For this review, take the finished solid that the model builds, in its own axes (mm). Give positions to 0.01 mm unless a question says otherwise; leave off trailing zeros. Order: outer loops, then holes, each group sorted by start corner. A loop starts at its lowest first (then second) coordinate and runs counter-clockwise, first axis right, second up.
Item 1: Consider section D-D (y = -63.5). Give the boundary of the cut face in (x, z) (3 decimals), plus the area to 3 significant figures.
Item 2: Consider section B-B (z = 1.45). Give the number of separate pieces and of enclosed holes in the cut face, plus the area to 3 significant figures.
Item 3: The part is to be moulded in two halves that separate along X. For faces 1 (the cylindrical face through (60.272, 21.508, 1.61)), 2 (the cylindrical face through (-22.79, 45.48, 1.61)), 3 (the flat face through (15.5, 1, 3.175)), 4 (the cylindrical face through (-58.958, -45.207, 1.565)), say which applies: released by +X, released by -X, zero draft, split by the parting line, or undercut.
Item 4: For probe 1 along X at (y, z) = (-58.42, 1.1); probe 2 along Y at (x, z) = (-60, 1.2), list the stretches that pass through material, from the lowest coordinate up.
Item 5: Consider section C-C (x = 45). Give the boundary of the cut face in (y, z) (3 decimals).
Item 6: For P1, Ø1.5, axis at y = 36, z = 2.5, coming from the -X side; P2, Ø1, axis at x = 28.5, z = 2.5, coming from the +Y side, all flat-tipped, find the tip position at first contact; note any pin that passes through.
Item 7: Consider section A-A (x = 0). Give the boundary of the cut face in (y, z) (1 decimal), plus the area to 3 significant figures.
```python
from build123d import *

# Parameters (mm, degrees)
F0_R            = 74.295
F1_DEPTH        = 3.175
F2_R            = 1.8542
F3_DEPTH        = 3.176
F3_COPIES_COUNT = 4
F4_R            = 14.9225
F4_R_2          = 3.302
F5_DEPTH        = 3.176
F6_R            = 1.8415
F7_DEPTH        = 3.176
F8_R            = 1.1303
F9_DEPTH        = 3.176


# Not quite as in the source:
# - a pattern or mirror of a feature is missing from the dataset's text; its kind, count and spacing are read off the source's solid


with BuildPart() as f1:
    # F0 (on Top) → F1 (new body)
    with BuildSketch(Plane.XY):
        Circle(F0_R)
    extrude(amount=F1_DEPTH)

    # F2 (on face) → F3 (cut, through all)
    with BuildSketch(Plane.XY.offset(3.175)):
        with BuildLine():
            ThreePointArc((-58.42, 19.7358), (-57.1088826063, 20.2788826063), (-56.5658, 21.59))
            ThreePointArc((-56.5658, 21.59), (-59.7311173937, 22.9011173937), (-58.42, 19.7358))
        make_face()
        with Locations((-58.42, -21.59)):
            Circle(F2_R)
    f3 = extrude(amount=-F3_DEPTH, mode=Mode.SUBTRACT)

    # F3_copies: F3 ×4 about axis
    f3_copies_axis = Axis((0, 0, 0), (0, 0, 1))
    for i in range(1, F3_COPIES_COUNT):
        add(f3.rotate(f3_copies_axis, i * 360 / F3_COPIES_COUNT), mode=Mode.SUBTRACT)

    # F4 (on face) → F5 (cut, through all)
    with BuildSketch(Plane.XY.offset(3.175)):
        Circle(F4_R)
        with Locations((-22.225, 0)):
            Circle(F4_R_2)
        with Locations((22.225, 0)):
            Circle(F4_R_2)
    extrude(amount=-F5_DEPTH, mode=Mode.SUBTRACT)

    # F6 (on face) → F7 (cut, through all)
    with BuildSketch(Plane.XY.offset(3.175)):
        with Locations((-21.330000012, 46.603412)):
            Circle(F6_R)
        with Locations((25.913999988, 46.603412)):
            Circle(F6_R)
        with Locations((5.593999988, -25.532588)):
            Circle(F6_R)
        with Locations((18.293999988, -25.532588)):
            Circle(F6_R)
    extrude(amount=-F7_DEPTH, mode=Mode.SUBTRACT)

    # F8 (on face) → F9 (cut, through all)
    with BuildSketch(Plane.XY.offset(3.175)):
        with Locations((-14.3844060319, 31.369)):
            Circle(F8_R)
        with Locations((-62.6444060319, -1.651)):
            Circle(F8_R)
        with Locations((-32.1644060319, -32.131)):
            Circle(F8_R)
    extrude(amount=-F9_DEPTH, mode=Mode.SUBTRACT)


solid = f1.part
```
Resolved:
1. outline: (-38.568, 0) - (38.568, 0) - (38.568, 3.175) - (-38.568, 3.175) - close
1. area: 245 mm2
2. separate pieces: 1
2. enclosed holes: 18
2. area: 16,400 mm2
3. face 1: undercut
3. face 2: undercut
3. face 3: zero draft
3. face 4: split by the parting line
4. probe 1: x = -45.9 to -23.44, -19.74 to 19.74, 23.44 to 45.9
4. probe 2: y = -43.81 to -22.56, -20.62 to 20.62, 22.56 to 43.81
5. outline: (-59.116, 0) - (59.116, 0) - (59.116, 3.175) - (-59.116, 3.175) - close
6. P1: stops at x = -65.4
6. P2: stops at y = 68.82
7. outline: (-74.3, 0) - (-14.9, 0) - (-14.9, 3.2) - (-74.3, 3.2) - close; (14.9, 0) - (74.3, 0) - (74.3, 3.2) - (14.9, 3.2) - close
7. area: 377 mm2
